Read the model definition and answer for the solid it produces. Units are mm, in the model's axes. A direction names the side the tool comes from. Give positions to 0.01 mm unless a question says otherwise; leave off trailing zeros. Order: outer loops, then holes, each group sorted by start corner. A loop starts at its lowest first (then second) coordinate and runs counter-clockwise, first axis right, second up. Notation, with made-up numbers: (-24.5, 69) - (17.5, 69) arc R10 ccw to (17.5, 78) - close; hole circle Ø2 at (78, -12). An arc over 180 degrees is marked (long way). Write each question's results on one line, items separated by ' | '. Start each with the question number.
Q1. For a pull along Z with two mould halves and no side action, classify faces 1 (the face through (8, -5, 5)), 2 (the face through (0.41, -0.12, 4.45)), 3 (the face through (8.692, -4.699, 0.285)) as +Z half, -Z half, draft (parallel to the pull), parting line (faces both ways), or undercut.
Q2. Find the intervals of material crossed by line 1 along Z through (x, y) = (5, 0); line 2 along Y through (x, z) = (13.25, 5); line 3 along Y through (x, z) = (10.5, 8.5), in increasing order. Write a range as from..to.
Q3. Flat-ended cylindrical pins translate along their axes: P1, Ø3, axis at x = -4.5, z = 6.5, coming from the +Y side; P2, Ø2, axis at x = -10.5, z = 6.5, coming from the +Y side; P3, Ø3, axis at x = 9, z = 2.5, coming from the +Y side; P4, Ø1.5, axis at y = 5.5, z = 4, coming from the +X side. Find the tip coordinate at first contact, or state that the pin passes through.
Q4. Find section A-A on x = 0.5. Give the vertices of the cut face in (y, z).
Q5. A tool of negligible diameter and unlimited length cuts with its end or side. For faces 4 (the face through (9.418, 0.423, 8.222)), 5 (the face through (8.455, 4.699, 0.285)), 6 (the face through (8.455, 4.699, 9.715)), from which of +Z, -Z, +X, -X, +Y, -Y can it reach the whole face along a straight path? Write none if from no direction.
from build123d import *

# Parameters (mm, degrees)
F0_R     = 2.75
F1_DEPTH = 10
F2_R     = 10
F3_R     = 1
F5_D     = 6.5
F5_DEPTH = 15
F5_TIP   = 1.9527970118


# Not quite as in the source:
# - a feature names something its author has since deleted; it is built from what else it names


with BuildPart() as f1:
    # F0 (on Top) → F1 (new body)
    with BuildSketch(Plane.XY):
        with BuildLine():
            ThreePointArc((-2.9769337647, -5), (-1.4225088619, -2.7117470016), (-0.8759132502, 0))
            ThreePointArc((-0.8759132502, 0), (-1.4225088619, 2.7117470016), (-2.9769337647, 5))
            ThreePointArc((-2.9769337647, 5), (-14.8759132502, 0), (-2.9769337647, -5))
        make_face()
        with Locations((-7.8759132502, 0)):
            Circle(F0_R, mode=Mode.SUBTRACT)
        with BuildLine():
            ThreePointArc((-2.9769337647, 5), (-1.4225088619, 2.7117470016), (-0.8759132502, 0))
            ThreePointArc((-0.8759132502, 0), (-1.4225088619, -2.7117470016), (-2.9769337647, -5))
            Line((-2.9769337647, -5), (17.0230662353, -5))
            Line((17.0230662353, -5), (17.0230662353, 5))
            Line((17.0230662353, 5), (-2.9769337647, 5))
        make_face()
    extrude(amount=F1_DEPTH)

    # F2
    f2_edges = [f1.edges().sort_by_distance(p)[0] for p in [
        (-2.976934, 5, 5),
        (-2.976934, -5, 5),
    ]]
    fillet(f2_edges, radius=F2_R)

    # F3
    f3_edges = [f1.edges().sort_by_distance(p)[0] for p in [
        (8.573576, 5, 10),
        (-2.30127, 5.298575, 10),
        (8.573576, 5, 0),
    ]]
    fillet(f3_edges, radius=F3_R)

    # F5
    with Locations(Plane.YZ.offset(17.0230662353)):
        with Locations((0, 5)):
            Hole(F5_D / 2, depth=F5_DEPTH)
            with Locations((0, 0, -(F5_DEPTH + F5_TIP / 2))):  # 118° drill point
                Cone(0, F5_D / 2, F5_TIP, mode=Mode.SUBTRACT)


solid = f1.part
Working result:
1) face 1: draft | face 2: undercut | face 3: -Z half
2) line 1: 0..1.75, 8.25..10 | line 2: -5..-3.25, 3.25..5 | line 3: -5..5
3) P1: y = 6.74 | P2: y = 6.81 | P3: y = 5 | P4: x = 17.02
4) outline: (-5, 1) arc R1 ccw to (-4, 0) - (4, 0) arc R1 ccw to (5, 1) - (5, 9) arc R1 ccw to (4, 10) - (-4, 10) arc R1 ccw to (-5, 9) - close; hole circle Ø1.43 at (0, 5)
5) face 4: +X | face 5: -Z, +X, +Y | face 6: +Z, +X, +Y
